Source: CAD feature listing. Evaluate the final solid. Frame: model axes, mm. Face numbers are marked on the shaded views. Give positions to 0.01 mm unless a question says otherwise; leave off trailing zeros. Order: outer loops, then holes, each group sorted by start corner. A loop starts at its lowest first (then second) coordinate and runs counter-clockwise, first axis right, second up.
```python
from build123d import *

# Parameters (mm, degrees)
SKETCH_1_R      = 26
SKETCH_2_R      = 16
SHELL_1_T       = -5
FILLET_1_R      = 10
SKETCH_4_R      = 22
EXTRUDE_1_DEPTH = 8
SKETCH_5_R      = 19.696379945
EXTRUDE_2_DEPTH = 12
FILLET_2_R      = 10
SKETCH_6_R      = 23.647308565
EXTRUDE_3_DEPTH = 0.8


with BuildPart() as part:
    # 草图1 → 放样1 section 0
    with BuildSketch(Plane.XY):
        Circle(SKETCH_1_R)
    # 草图2 → 放样1 section 1
    with BuildSketch(Plane.XY.offset(-11)):
        Circle(SKETCH_2_R)
    loft()

    # 抽壳1
    shell_1_openings = [part.faces().sort_by_distance(p)[0] for p in [
        (0, 0, 0),
    ]]
    offset(amount=SHELL_1_T, openings=shell_1_openings, kind=Kind.INTERSECTION)

    # 圆角1
    fillet_1_edges = [part.edges().sort_by_distance(p)[0] for p in [
        (-13.788150569, 0, -6),
    ]]
    fillet(fillet_1_edges, radius=FILLET_1_R)

    # 草图3 → 旋转1 (revolve)
    with BuildSketch(Plane(origin=(0, 0, 0), x_dir=(1, 0, 0), z_dir=(0, 1, 0)), mode=Mode.PRIVATE) as revolve_1_sk:
        with BuildLine():
            Line((0, 6), (6.731942195, 6))
            ThreePointArc((6.731942195, 6), (4.217222472, 2.331539651), (0, 0.91858132))
            Line((0, 0.91858132), (0, 6))
        make_face()
    revolve(revolve_1_sk.sketch.rotate(Axis((0, 0, 7.141645332), (0, 0, -1)), 180), axis=Axis((0, 0, 7.141645332), (0, 0, -1)))

    # 草图4 → 拉伸1 (add)
    with BuildSketch(Plane(origin=(0, 0, -11), x_dir=(-1, 0, 0), z_dir=(0, 0, -1))):
        Circle(SKETCH_4_R)
    extrude(amount=EXTRUDE_1_DEPTH)

    # 草图5 → 拉伸2 (add)
    with BuildSketch(Plane(origin=(0, 0, -21), x_dir=(-1, 0, 0), z_dir=(0, 0, -1))):
        Circle(SKETCH_5_R)
    extrude(amount=-EXTRUDE_2_DEPTH)

    # 圆角2
    fillet_2_edges = [part.edges().sort_by_distance(p)[0] for p in [
        (-19.242696024, 0, 0),
    ]]
    fillet(fillet_2_edges, radius=FILLET_2_R)

    # 草图6 → 拉伸3 (add)
    with BuildSketch(Plane.XY):
        with BuildLine():
            Line((-3.856946079, 36.181818182), (-20.056119612, 16.545454545))
            ThreePointArc((-20.056119612, 16.545454545), (-26, 0), (-20.056119612, -16.545454545))
            Line((-20.056119612, -16.545454545), (-3.856946079, -36.181818182))
            ThreePointArc((-3.856946079, -36.181818182), (0, -38), (3.856946079, -36.181818182))
            Line((3.856946079, -36.181818182), (20.056119612, -16.545454545))
            ThreePointArc((20.056119612, -16.545454545), (26, 0), (20.056119612, 16.545454545))
            Line((20.056119612, 16.545454545), (3.856946079, 36.181818182))
            ThreePointArc((3.856946079, 36.181818182), (0, 38), (-3.856946079, 36.181818182))
        make_face()
        Circle(SKETCH_6_R, mode=Mode.SUBTRACT)
        with BuildLine():
            Line((-2, 34), (-2, 32))
            ThreePointArc((-2, 32), (0, 30), (2, 32))
            Line((2, 32), (2, 34))
            ThreePointArc((2, 34), (0, 36), (-2, 34))
        make_face(mode=Mode.SUBTRACT)
        with BuildLine():
            Line((2, -34), (2, -32))
            ThreePointArc((2, -32), (0, -30), (-2, -32))
            Line((-2, -32), (-2, -34))
            ThreePointArc((-2, -34), (0, -36), (2, -34))
        make_face(mode=Mode.SUBTRACT)
    extrude(amount=-EXTRUDE_3_DEPTH)


solid = part.part
```
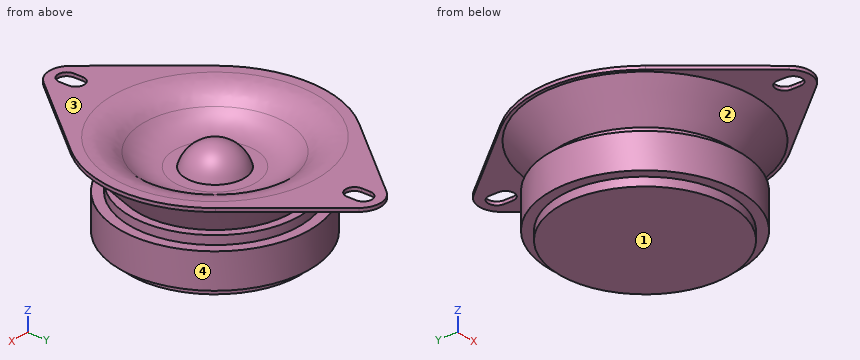
1) Pin query (flat end, axial travel): pin 1 (5 mm diameter, centred on x = -13, y = 3, fed in from +Z); pin 2 (3 mm diameter, centred on y = 21, z = -17.5, fed in from +X); pin 3 (8 mm diameter, centred on y = -12, z = -9.5, fed in from +X). Return the tip coordinate at first contact, or that it passes through.
Report:
pin 1: stops at z = -3.62
pin 2: stops at x = 10.19
pin 3: stops at x = 20.38
2) Material intervals for L1, parallel to Y at x = 2.5, z = -4; L2, parallel to Z at x = -8, y = 0.5; L3, parallel to Z at x = 6, y = -28, sorted ascending.
Report:
L1: y = -22.22 to -15.16, -5.23 to 5.23, 15.16 to 22.22
L2: z = -21 to -6
L3: z = -0.8 to 0
3) Draft query along Z for the marked faces 1, 2, 3 and 4. Return one class per face: +Z half, -Z half, draft (parallel to the pull), parting line (faces both ways), or undercut.
Report:
face 1: -Z half
face 2: undercut
face 3: +Z half
face 4: draft
4) Section query A-A, the plane z = -12.5. Return the cut outline in (x, y), and give its area (3 significant figures).
Report:
outline: circle Ø44 at (0, 0)
area: 1,520 mm2
